Geometry: final body of the model. Coordinates: model frame, mm. A direction names the side the tool comes from. Give positions to 0.01 mm unless a question says otherwise; leave off trailing zeros. Write each loop counter-clockwise with the first axis right and the second up, starting at its lowest first coordinate (ties: lowest second). Pieces come first, ordered by that corner, then holes. Notation, with made-up numbers: M 68.25,-34.5 L 113.25,-34.5 A29 cw 113.25,-9.5 Z; hole C 30.25,-2.75 d5. An arc over 180 degrees is marked long. Answer as a JSON object with one key per item and string values.
from build123d import *

# Parameters (mm, degrees)
F0_R     = 9.652
F0_R_2   = 3.8735
F1_DEPTH = 2.54
F2_R     = 4.0005
F3_DEPTH = 6.096
F4_R     = 2.54
F5_DEPTH = 4.572


with BuildPart() as f1:
    # F0 (on Top) → F1 (new body)
    with BuildSketch(Plane.XY):
        Circle(F0_R)
        Circle(F0_R_2, mode=Mode.SUBTRACT)
    extrude(amount=F1_DEPTH)

    # F2 (on Top) → F3 (join)
    with BuildSketch(Plane.XY):
        Circle(F2_R)
    extrude(amount=F3_DEPTH)

    # F4 (on face) → F5 (cut)
    with BuildSketch(Plane.XY.offset(6.096)):
        Circle(F4_R)
    extrude(amount=-F5_DEPTH, mode=Mode.SUBTRACT)


solid = f1.part
1) Line query: line 1 (Y direction, x = 0, z = 3.6); line 2 (Z direction, x = -3.75, y = 2); line 3 (X direction, y = 1.5, z = 4.75). Output: solid intervals per line, ascending. Write a range as from..to.
Geometry check:
{"line 1": "y = -4..-2.54, 2.54..4", "line 2": "z = 0..2.54", "line 3": "x = -3.71..-2.05, 2.05..3.71"}
2) Cut plane B-B on z = 3. Return loops of the section in (x, y).
Geometry check:
{"outline": "C 0,0 d8; hole C 0,0 d5.08"}
3) Set-up query: faces 4 (the flat face through (4.2, 0.1, 2.54)), 5 (the flat face through (3, 0, 6.096)). Return all of +Z, -Z, +X, -X, +Y, -Y with unobstructed straight access to the full face (end or side cutting, diameter ignored); none if empty.
Geometry check:
{"face 4": "+Z", "face 5": "+Z, +X, -X, +Y, -Y"}
4) Pull-direction query (Y, two-part tool) for faces 1 (the flat face through (0, 0, 1.524)), 2 (the cylindrical face through (-0.9, -3.9, 4.3)), 3 (the flat face through (0, 0, 0)); classes: pulls with the +Y half, pulls with the -Y half, needs draft (parallel to the pull), parting line crosses it, or undercut.
Geometry check:
{"face 1": "undercut", "face 2": "parting line crosses it", "face 3": "needs draft"}
5) Contact query for flat-ended pins moving along their axis: P1, Ø2.5, axis at x = 0.5, y = -1, coming from the +Z side; P2, Ø1.5, axis at y = -2, z = 3.5, coming from the -X side; P3, Ø6, axis at x = 6, y = 5.5, coming from the +Z side. Output: stop coordinate, or through.
Geometry check:
{"P1": "stops at z = 1.52", "P2": "stops at x = -3.8", "P3": "stops at z = 2.54"}
6) Cut plane D-D on x = -8. Return loops of the section in (y, z).
Geometry check:
{"outline": "M -5.4,0 L 5.4,0 L 5.4,2.54 L -5.4,2.54 Z"}
7) Cut plane A-A on y = 0. Return loops of the section in (x, z), and give its area (3 significant figures).
Geometry check:
{"outline": "M -9.65,0 L 9.65,0 L 9.65,2.54 L 4,2.54 L 4,6.1 L 2.54,6.1 L 2.54,1.52 L -2.54,1.52 L -2.54,6.1 L -4,6.1 L -4,2.54 L -9.65,2.54 Z", "area": "54.3 mm2"}
